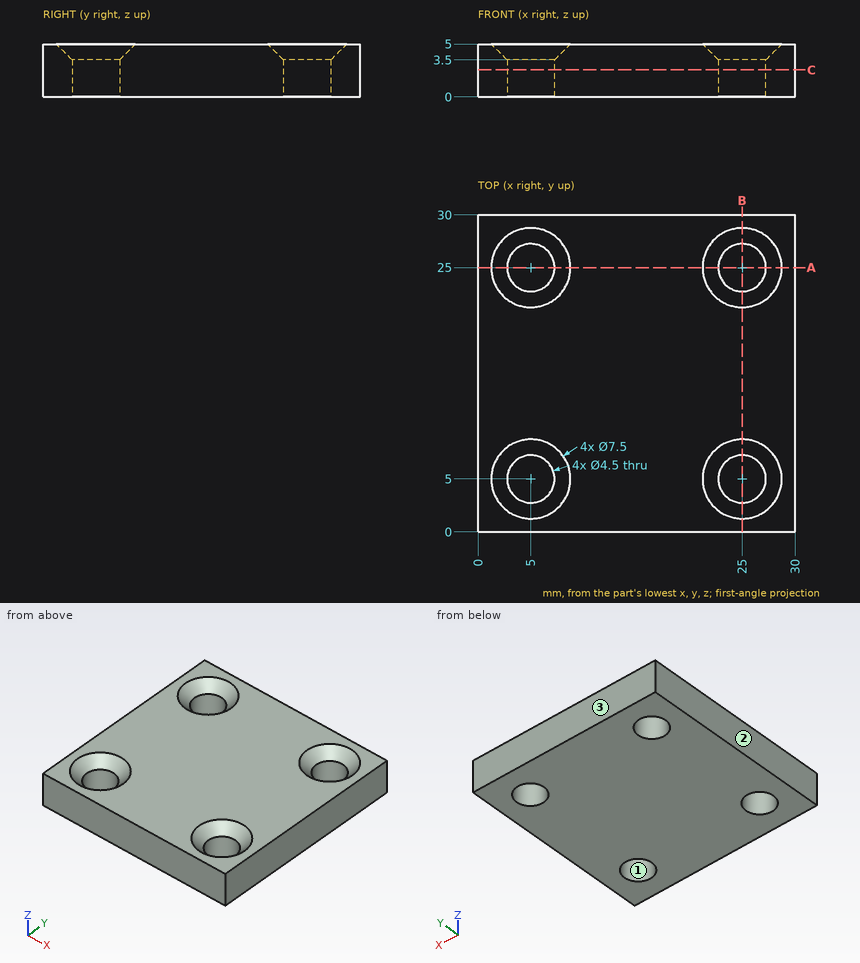
Answer from the drawing. Dimensions are ordinates in mm from the lowest x, y and z of the part. Give positions to 0.01 mm unless a question says otherwise; leave off trailing zeros. Order: outer loops, then holes, each group sorted by start corner. A loop starts at its lowest first (then second) coordinate and runs counter-clockwise, first axis right, second up.
(1) Straight lines are drawn through the part: L1, parallel to Y at x = 5, z = 2.15; L2, parallel to Y at x = 26.75, z = 2.9; L3, parallel to X at y = 3.75, z = 3.6. For each, find the intervals that lie inside material, in ascending order.
(2) Given pin 1 (7 mm diameter, centred on x = 25, y = 5, fed in from +Z); pin 2 (6 mm diameter, centred on x = 25, y = 25, fed in from -Z), each flat-ended and moving along its own axis, determine where each tip first touches the part or whether it passes through.
(3) Find section C-C (z = 2.55). Give the vertices of the cut face in (x, y).
(4) Find section A-A (y = 25). Give the vertices of the cut face in (x, z).
(5) For a pull along Y with two mould halves and no side action, classify the marked faces 1, 2 and 3 as released by +Y, released by -Y, zero draft, split by the parting line, or undercut.
Result sheet:
1. L1: y = 0 to 2.75, 7.25 to 22.75, 27.25 to 30
1. L2: y = 0 to 3.59, 6.41 to 23.59, 26.41 to 30
1. L3: x = 0 to 3.01, 6.99 to 23.01, 26.99 to 30
2. pin 1: stops at z = 4.75
2. pin 2: stops at z = 0
3. outline: (0, 0) - (30, 0) - (30, 30) - (0, 30) - close; hole circle Ø4.5 at (5, 5); hole circle Ø4.5 at (5, 25); hole circle Ø4.5 at (25, 5); hole circle Ø4.5 at (25, 25)
4. outline: (0, 0) - (2.75, 0) - (2.75, 3.5) - (1.25, 5) - (0, 5) - close; (7.25, 0) - (22.75, 0) - (22.75, 3.5) - (21.25, 5) - (8.75, 5) - (7.25, 3.5) - close; (27.25, 0) - (30, 0) - (30, 5) - (28.75, 5) - (27.25, 3.5) - close
5. face 1: undercut
5. face 2: zero draft
5. face 3: released by +Y
